For this review, take the finished solid that the model builds, in its own axes (mm). Coordinates: 2 decimals unless noted, no trailing zeros. Order: outer loops, then holes, each group sorted by start corner. A loop starts at its lowest first (then second) coordinate and runs counter-clockwise, first axis right, second up.
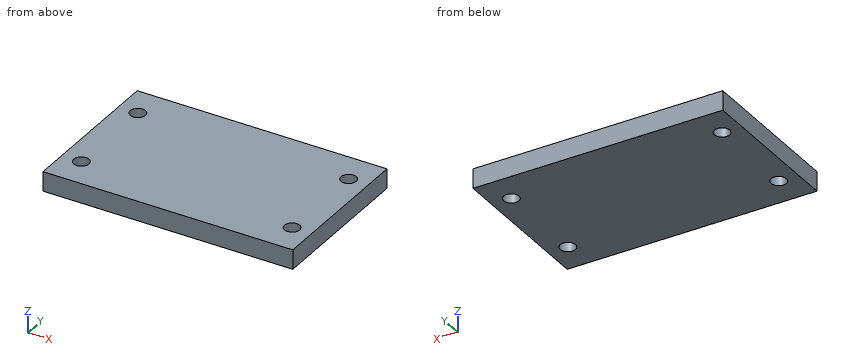
from build123d import *

# Parameters (mm, degrees)
F0_W     = 81.28
F0_H     = 50.8
F1_DEPTH = 6.35
F2_D     = 4.9784


with BuildPart() as f1:
    # F0 (on Top) → F1 (new body)
    with BuildSketch(Plane.XY):
        with Locations((-106.3625, 0)):
            Rectangle(F0_W, F0_H)
    extrude(amount=-F1_DEPTH)

    # F2 (through all)
    with Locations(Plane.XY):
        with Locations((-140.6525, 15.24), (-140.6525, -15.24), (-72.0725, 15.24), (-72.0725, -15.24)):
            Hole(F2_D / 2)


solid = f1.part
1. To check wall thickness, follow L1, parallel to X at y = -15, z = -0.5; L2, parallel to X at y = -13, z = -0.75; L3, parallel to Y at x = -139, z = -5.5. State the ranges of each line that lie inside material, in increasing order.
Answer below:
L1: x = -147 to -143.13, -138.17 to -74.55, -69.59 to -65.72
L2: x = -147 to -141.74, -139.57 to -73.16, -70.99 to -65.72
L3: y = -25.4 to -17.1, -13.38 to 13.38, 17.1 to 25.4
2. Take a section at B-B, the plane z = -3. Give the boundary of the cut face in (x, y), plus the area to 3 significant figures.
Answer below:
outline: (-147, -25.4) - (-65.72, -25.4) - (-65.72, 25.4) - (-147, 25.4) - close; hole circle Ø4.98 at (-140.65, -15.24); hole circle Ø4.98 at (-140.65, 15.24); hole circle Ø4.98 at (-72.07, -15.24); hole circle Ø4.98 at (-72.07, 15.24)
area: 4,050 mm2
3. Take a section at C-C, the plane x = -139. Give the boundary of the cut face in (y, z), plus the area to 3 significant figures.
Answer below:
outline: (-25.4, -6.35) - (-17.1, -6.35) - (-17.1, 0) - (-25.4, 0) - close; (-13.38, -6.35) - (13.38, -6.35) - (13.38, 0) - (-13.38, 0) - close; (17.1, -6.35) - (25.4, -6.35) - (25.4, 0) - (17.1, 0) - close
area: 275 mm2
4. Take a section at A-A, the plane y = 15.24. Give the boundary of the cut face in (x, z).
Answer below:
outline: (-147, -6.35) - (-143.14, -6.35) - (-143.14, 0) - (-147, 0) - close; (-138.16, -6.35) - (-74.56, -6.35) - (-74.56, 0) - (-138.16, 0) - close; (-69.58, -6.35) - (-65.72, -6.35) - (-65.72, 0) - (-69.58, 0) - close
